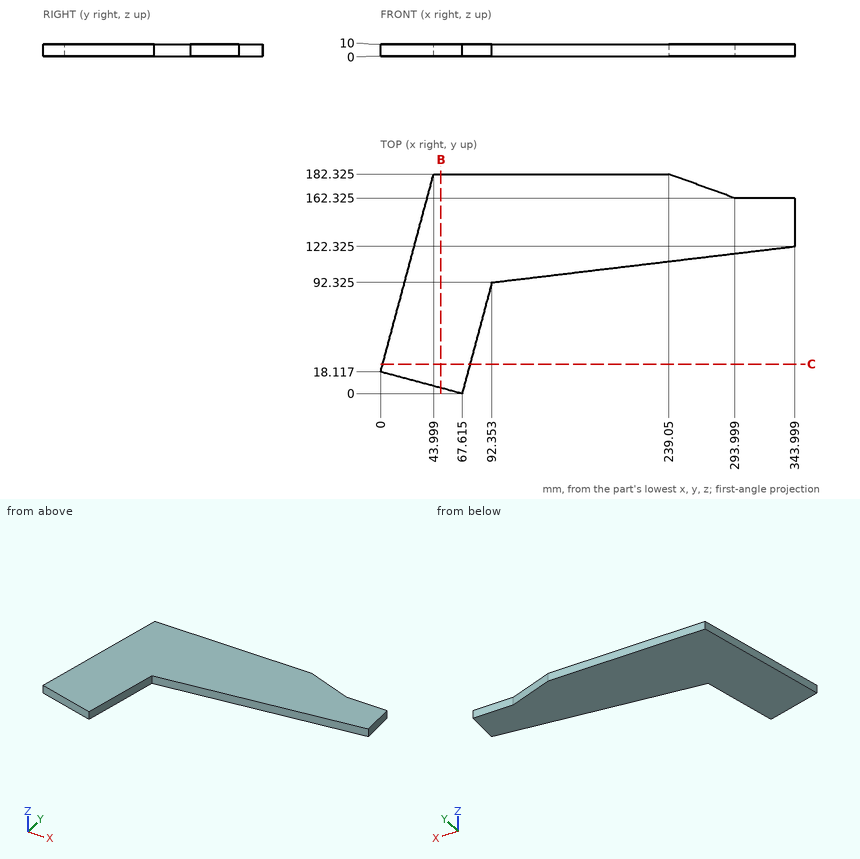
Here's the drawing with two shaded views (mm, measured from the low corner). I have some questions. Give positions to 0.01 mm unless a question says otherwise; leave off trailing zeros. Write each loop counter-clockwise with the first axis right and the second up, starting at its lowest first coordinate (ties: lowest second). Pieces come first, ordered by that corner, then holes. Notation, with made-up numbers: (64, -18.75) - (121, -18.75) arc R11 ccw to (121, -7.75) - close; hole circle Ø3 at (72, 3.5). An arc over 180 degrees is marked (long way). Write item = value, one per line. Start each with the question number.
1. Please list where these lines run through material, in increasing order: line 1 (Y direction, x = 208.5, z = 3.75) (1 decimal); line 2 (X direction, y = 160, z = 2); line 3 (X direction, y = 20, z = 9) (1 decimal).
2. Imagine slicing it at C-C (y = 24.5). Please give me the cut outline in (x, z).
3. Imagine slicing it at B-B (x = 50). Please give me the cut outline in (y, z) (1 decimal), and give its area (3 significant figures).
4. For pin 1 (3 mm diameter, centred on x = 119.5, z = 8, fed in from -Y); pin 2 (3 mm diameter, centred on y = 83, z = 6.5, fed in from -X); pin 3 (5 mm diameter, centred on y = 28.5, z = 7, fed in from +X), each with a flat end and sliding along its axis, tell me the tip position at first contact or that it passes through.
Worked answers:
q1.line_1 = 106.2 to 182.3
q1.line_2 = 38.02 to 344
q1.line_3 = 0.5 to 73
q2.outline = (1.71, 0) - (74.18, 0) - (74.18, 10) - (1.71, 10) - close
q3.outline = (4.7, 0) - (182.3, 0) - (182.3, 10) - (4.7, 10) - close
q3.area = 1,780 mm2
q4.pin_1 = 95.38
q4.pin_2 = 16.98
q4.pin_3 = 75.92
